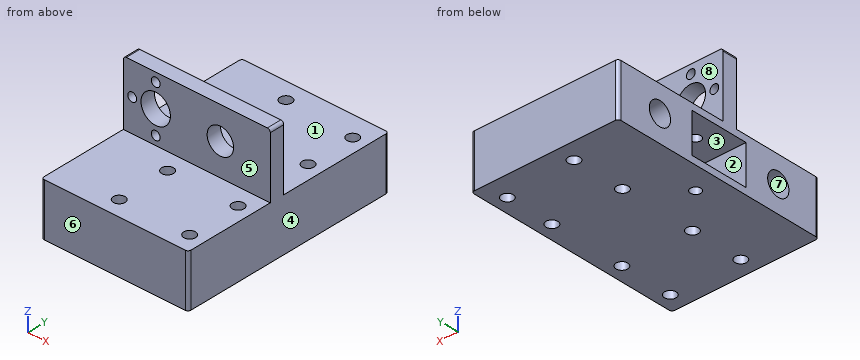
from build123d import *

# Parameters (mm, degrees)
SKETCH1_W           = 50
SKETCH1_H           = 74
SKETCH1_R           = 2
BOSS_EXTRUDE1_DEPTH = 18
SKETCH5_W           = 50
SKETCH5_H           = 18
BOSS_EXTRUDE3_DEPTH = 5.5
SKETCH7_W           = 50
SKETCH7_H           = 5
BOSS_EXTRUDE5_DEPTH = 22
CUT_EXTRUDE1_REACH  = 94.441
SKETCH8_R           = 4.5
SKETCH8_R_2         = 5
SKETCH10_R          = 3.95
SKETCH10_W          = 13.5
SKETCH10_H          = 20
CUT_EXTRUDE2_DEPTH  = 20
CUT_EXTRUDE3_REACH  = 55.993
SKETCH11_R          = 1.75
FILLET2_R           = 1
BOSS_EXTRUDE6_START = -44
SKETCH12_R          = 5
SKETCH12_R_2        = 4.5
BOSS_EXTRUDE6_DEPTH = 5
CUT_EXTRUDE4_REACH  = 65.492
FILLET3_R           = 1
CUT_EXTRUDE5_REACH  = 63.205
SKETCH14_R          = 1.5


with BuildPart() as part:
    # Sketch1 → Boss-Extrude1 (new body)
    with BuildSketch(Plane.XY):
        Rectangle(SKETCH1_W, SKETCH1_H)
        with Locations((-4, 31)):
            Circle(SKETCH1_R, mode=Mode.SUBTRACT)
        with Locations((20, 29.6)):
            Circle(SKETCH1_R, mode=Mode.SUBTRACT)
        with Locations((20, 13)):
            Circle(SKETCH1_R, mode=Mode.SUBTRACT)
        with Locations((-4, 13)):
            Circle(SKETCH1_R, mode=Mode.SUBTRACT)
        with Locations((-4, -13)):
            Circle(SKETCH1_R, mode=Mode.SUBTRACT)
        with Locations((20, -13)):
            Circle(SKETCH1_R, mode=Mode.SUBTRACT)
        with Locations((20, -31)):
            Circle(SKETCH1_R, mode=Mode.SUBTRACT)
        with Locations((-4, -31)):
            Circle(SKETCH1_R, mode=Mode.SUBTRACT)
    extrude(amount=BOSS_EXTRUDE1_DEPTH)

    # Sketch5 → Boss-Extrude3 (add)
    with BuildSketch(Plane(origin=(0, 37, 0), x_dir=(1, 0, 0), z_dir=(0, 1, 0))):
        with Locations((0, -9)):
            Rectangle(SKETCH5_W, SKETCH5_H)
    extrude(amount=BOSS_EXTRUDE3_DEPTH)

    # Sketch7 → Boss-Extrude5 (add)
    with BuildSketch(Plane.XY.offset(18)):
        with Locations((0, 40)):
            Rectangle(SKETCH7_W, SKETCH7_H)
    extrude(amount=BOSS_EXTRUDE5_DEPTH)

    # Sketch8 → Cut-Extrude1 (cut, up to next)
    with BuildSketch(Plane(origin=(0, 42.5, 0), x_dir=(1, 0, 0), z_dir=(0, 1, 0)), mode=Mode.PRIVATE) as cut_extrude1_sk1:
        with Locations(Location((8, -29, 0), (0, 0, 270))):
            Circle(SKETCH8_R)
    cut_extrude1_tool1 = extrude(cut_extrude1_sk1.sketch, amount=-CUT_EXTRUDE1_REACH, mode=Mode.PRIVATE) & part.part
    # Sketch8 → Cut-Extrude1 (cut, up to next)
    with BuildSketch(Plane(origin=(0, 42.5, 0), x_dir=(1, 0, 0), z_dir=(0, 1, 0)), mode=Mode.PRIVATE) as cut_extrude1_sk2:
        with Locations(Location((-14, -29, 0), (0, 0, 270))):
            Circle(SKETCH8_R_2)
    cut_extrude1_tool2 = extrude(cut_extrude1_sk2.sketch, amount=-CUT_EXTRUDE1_REACH, mode=Mode.PRIVATE) & part.part
    add(cut_extrude1_tool1.solids().sort_by_distance((8, 42.5, 29))[0], mode=Mode.SUBTRACT)
    add(cut_extrude1_tool2.solids().sort_by_distance((-14, 42.5, 29))[0], mode=Mode.SUBTRACT)

    # Sketch10 → Cut-Extrude2 (cut)
    with BuildSketch(Plane.ZY.offset(25)):
        with Locations((9, 22)):
            Circle(SKETCH10_R)
        with Locations((9, -22)):
            Circle(SKETCH10_R)
        with Locations((9, 0)):
            Rectangle(SKETCH10_W, SKETCH10_H)
    extrude(amount=-CUT_EXTRUDE2_DEPTH, mode=Mode.SUBTRACT)

    # Cut-Extrude3: up to this face of the body (flat: up to its plane)
    cut_extrude3_end = Plane(part.part.faces().sort_by_distance((-0.207576241, 2.825895063, 0))[0])
    # Sketch11 → Cut-Extrude3 (cut, up to the picked face)
    with BuildSketch(Plane.XY.offset(18), mode=Mode.PRIVATE) as cut_extrude3_sk1:
        with Locations(Location((-17, 0, 0), (0, 0, 180))):
            Circle(SKETCH11_R)
    cut_extrude3_tool1 = split(extrude(cut_extrude3_sk1.sketch, amount=-CUT_EXTRUDE3_REACH, mode=Mode.PRIVATE), bisect_by=cut_extrude3_end, keep=Keep.BOTH, mode=Mode.PRIVATE)
    add(cut_extrude3_tool1.solids().sort_by(Axis((-17, 0, 18), (0, 0, -1)))[0], mode=Mode.SUBTRACT)

    # Fillet2
    fillet2_edges = [part.edges().sort_by_distance(p)[0] for p in [
        (25, 42.5, 20),
        (-25, 42.5, 20),
        (25, -37, 9),
        (-25, -37, 9),
    ]]
    fillet(fillet2_edges, radius=FILLET2_R)

    # Sketch12 → Boss-Extrude6 (add)
    with BuildSketch(Plane(origin=(0, 42.5, 0), x_dir=(1, 0, 0), z_dir=(0, 1, 0)).offset(BOSS_EXTRUDE6_START)):
        Polygon((24, -40), (25, -40), (25, -18), (-25, -18), (-25, -40), (-24, -40), align=None)
        with Locations(Location((-14, -29, 0), (0, 0, 270))):
            Circle(SKETCH12_R, mode=Mode.SUBTRACT)
        with Locations(Location((8, -29, 0), (0, 0, 270))):
            Circle(SKETCH12_R_2, mode=Mode.SUBTRACT)
    extrude(amount=-BOSS_EXTRUDE6_DEPTH)

    # Sketch13 → Cut-Extrude4 (cut, up to next)
    with BuildSketch(Plane.XY.offset(40), mode=Mode.PRIVATE) as cut_extrude4_sk1:
        with BuildLine():
            Line((25, 37.5), (25, 41.5))
            ThreePointArc((25, 41.5), (24.707106781, 42.207106781), (24, 42.5))
            Line((24, 42.5), (-24, 42.5))
            ThreePointArc((-24, 42.5), (-24.707106781, 42.207106781), (-25, 41.5))
            Line((-25, 41.5), (-25, 37.5))
            Line((-25, 37.5), (25, 37.5))
        make_face()
    cut_extrude4_tool1 = extrude(cut_extrude4_sk1.sketch, amount=-CUT_EXTRUDE4_REACH, mode=Mode.PRIVATE) & part.part
    add(cut_extrude4_tool1.solids().sort_by_distance((0, 39.996085, 40))[0], mode=Mode.SUBTRACT)

    # Fillet3
    fillet3_edges = [part.edges().sort_by_distance(p)[0] for p in [
        (25, -4, 40),
        (-25, -4, 40),
        (25, 37.5, 9),
        (-25, 37.5, 9),
    ]]
    fillet(fillet3_edges, radius=FILLET3_R)

    # Sketch14 → Cut-Extrude5 (cut, up to next)
    with BuildSketch(Plane(origin=(0, -1.5, 0), x_dir=(1, 0, 0), z_dir=(0, 1, 0)), mode=Mode.PRIVATE) as cut_extrude5_sk1:
        with Locations(Location((-14, -21, 0), (0, 0, 270))):
            Circle(SKETCH14_R)
    cut_extrude5_tool1 = extrude(cut_extrude5_sk1.sketch, amount=-CUT_EXTRUDE5_REACH, mode=Mode.PRIVATE) & part.part
    # Sketch14 → Cut-Extrude5 (cut, up to next)
    with BuildSketch(Plane(origin=(0, -1.5, 0), x_dir=(1, 0, 0), z_dir=(0, 1, 0)), mode=Mode.PRIVATE) as cut_extrude5_sk2:
        with Locations(Location((-22, -29, 0), (0, 0, 270))):
            Circle(SKETCH14_R)
    cut_extrude5_tool2 = extrude(cut_extrude5_sk2.sketch, amount=-CUT_EXTRUDE5_REACH, mode=Mode.PRIVATE) & part.part
    # Sketch14 → Cut-Extrude5 (cut, up to next)
    with BuildSketch(Plane(origin=(0, -1.5, 0), x_dir=(1, 0, 0), z_dir=(0, 1, 0)), mode=Mode.PRIVATE) as cut_extrude5_sk3:
        with Locations(Location((-14, -37, 0), (0, 0, 270))):
            Circle(SKETCH14_R)
    cut_extrude5_tool3 = extrude(cut_extrude5_sk3.sketch, amount=-CUT_EXTRUDE5_REACH, mode=Mode.PRIVATE) & part.part
    add(cut_extrude5_tool1.solids().sort_by_distance((-14, -1.5, 21))[0], mode=Mode.SUBTRACT)
    add(cut_extrude5_tool2.solids().sort_by_distance((-22, -1.5, 29))[0], mode=Mode.SUBTRACT)
    add(cut_extrude5_tool3.solids().sort_by_distance((-14, -1.5, 37))[0], mode=Mode.SUBTRACT)


solid = part.part
Could you check a few things on this model? Use its own coordinates, in mm. Face numbers are marked on the shaded views. A direction names the side the tool comes from. Round coordinates to 2 decimals unless told otherwise and drop trailing zeros. Write each loop counter-clockwise with the first axis right and the second up, starting at its lowest first coordinate (ties: lowest second). Pieces come first, ordered by that corner, then holes. Notation, with made-up numbers: (37, 52) - (73, 52) arc R29 cw to (73, 85) - close; hole circle Ø5 at (48.5, 40.25). An arc over 180 degrees is marked (long way). Use a Markdown table: item, result.
Q1. Please list where these lines run through material, in increasing order: L1, parallel to Y at x = -4, z = 14.75; L2, parallel to X at y = -3, z = 29; L3, parallel to Y at x = -8.5, z = 14.5.
Output values:
| item | result |
|---|---|
| L1 | -37 to -33, -29 to -15, -11 to 11, 15 to 29, 33 to 37.5 |
| L2 | -25 to -23.5, -20.5 to -19, -9 to 3.5, 12.5 to 25 |
| L3 | -37 to -10, 10 to 37.5 |
Q2. I want a section at B-B (x = 20). List the corners of the cut face in (y, z) for me.
Output values:
| item | result |
|---|---|
| outline | (-37, 0) - (-33, 0) - (-33, 18) - (-37, 18) - close; (-29, 0) - (-15, 0) - (-15, 18) - (-29, 18) - close; (-11, 0) - (11, 0) - (11, 18) - (-1.5, 18) - (-1.5, 40) - (-6.5, 40) - (-6.5, 18) - (-11, 18) - close; (15, 0) - (27.6, 0) - (27.6, 18) - (15, 18) - close; (31.6, 0) - (37.5, 0) - (37.5, 18) - (31.6, 18) - close |
Q3. I want a section at D-D (y = -31). List the corners of the cut face in (x, z) for me, plus the area to 3 significant figures.
Output values:
| item | result |
|---|---|
| outline | (-25, 0) - (-6, 0) - (-6, 18) - (-25, 18) - close; (-2, 0) - (18, 0) - (18, 18) - (-2, 18) - close; (22, 0) - (25, 0) - (25, 18) - (22, 18) - close |
| area | 756 mm2 |
Q4. Thinking about a two-plate mould opening in Z: for the marked faces 1, 2, 3 and 4, which applies, released by +Z, released by -Z, zero draft, split by the parting line, or undercut?
Output values:
| item | result |
|---|---|
| face 1 | released by +Z |
| face 2 | undercut |
| face 3 | undercut |
| face 4 | zero draft |
Q5. I want a section at C-C (z = 29). List the corners of the cut face in (x, y) for me.
Output values:
| item | result |
|---|---|
| outline | (-25, -6.5) - (-23.5, -6.5) - (-23.5, -1.5) - (-25, -1.5) - close; (-20.5, -6.5) - (-19, -6.5) - (-19, -1.5) - (-20.5, -1.5) - close; (-9, -6.5) - (3.5, -6.5) - (3.5, -1.5) - (-9, -1.5) - close; (12.5, -6.5) - (25, -6.5) - (25, -1.5) - (12.5, -1.5) - close |
Q6. For pin 1 (24.5 mm diameter, centred on x = -1, y = -26, fed in from +Z); pin 2 (2.5 mm diameter, centred on x = -14, z = 21, fed in from +Y); pin 3 (4 mm diameter, centred on y = 3, z = 6.5, fed in from -X), each with a flat end and sliding along its axis, tell me the tip position at first contact or that it passes through.
Output values:
| item | result |
|---|---|
| pin 1 | z = 18 |
| pin 2 | through |
| pin 3 | x = -5 |
Q7. For the marked faces 5, 6, 7 and 8, which set-ups out of +Z, -Z, +X, -X, +Y, -Y let a thin tool reach every point of the face, with its end or its side?
Output values:
| item | result |
|---|---|
| face 5 | +Z, +X, -X, -Y |
| face 6 | +Z, -Z, +X, -X, -Y |
| face 7 | -X |
| face 8 | +Z, +X, -X, +Y |
Q8. I want a section at A-A (x = -17). List the corners of the cut face in (y, z) for me, plus the area to 3 significant figures.
Output values:
| item | result |
|---|---|
| outline | (-37, 0) - (-1.75, 0) - (-1.75, 2.25) - (-10, 2.25) - (-10, 15.75) - (-1.75, 15.75) - (-1.75, 18) - (-1.5, 18) - (-1.5, 25) - (-6.5, 25) - (-6.5, 18) - (-37, 18) - close; (-6.5, 33) - (-1.5, 33) - (-1.5, 40) - (-6.5, 40) - close; (1.75, 0) - (37.5, 0) - (37.5, 18) - (1.75, 18) - (1.75, 15.75) - (10, 15.75) - (10, 2.25) - (1.75, 2.25) - close; hole circle Ø7.9 at (-22, 9); hole circle Ø7.9 at (22, 9) |
| area | 1,030 mm2 |
